Autodesk Inventor part; units mm, degrees
ref_plane "YZ Plane" through (0, 0, 0) normal (1, 0, 0) x (0, 1, 0)
ref_plane "XZ Plane" through (0, 0, 0) normal (0, 1, 0) x (-1, 0, 0)
ref_plane "XY Plane" through (0, 0, 0) normal (0, 0, 1) x (1, 0, 0)
sketch "Skizze1" plane through (0, 0, 0) normal (0, 0, 1) x (1, 0, 0)
  line L0 (-210, 0) -> (210, 0)
  line L1 (0, -168) -> (0, 168)
  ellipse E0 centre (0, 0) end of major axis (-150, 0) minor radius 120
  line L2 (0, 120) -> (0, -120) construction
  line L3 (-150, 0) -> (150, 0) construction
  dimension "d0" = 300
  dimension "d1" = 240
extrude "Extrusion1" add sketch "Skizze1" along normal blind 10
sketch "Skizze2" plane through (0, 0, 10) normal (0, 0, 1) x (1, 0, 0)
  ellipse E0 centre (0, 0) end of major axis (-150, 0) minor radius 120
  line L0 (0, -168) -> (0, 168)
  line L1 (-210, 0) -> (210, 0)
  line L2 (-131.5, 0) -> (131.5, 0)
  line L3 (0, 101.5) -> (0, -101.5)
  ellipse E1 centre (0, 0) end of major axis (-131.5, 0) minor radius 101.5
  line L4 (0, 0) -> (-105.3012, -60.7957) construction
  line L5 (0, 0) -> (105.3012, -60.7957) construction
  ellipse E2 centre (0, 0) end of major axis (118.5, 0) minor radius 88.5
  line L6 (0, 0) -> (80.349, 80.349) construction
  line L7 (80.349, 80.349) -> (73.764, 69.2632)
  line L8 (67.3414, 73.0783) -> (84.3123, 62.9974)
  arc A0 (94.9826, -52.9176) -> (105.1165, -60.6891) centre (99.5391, -57.469) ccw
  arc A1 (-105.1165, -60.6891) -> (-94.9826, -52.9176) centre (-99.5391, -57.469) ccw
  point P0 (0, 120)
  point P1 (150, 0)
  point P2 (-150, 0)
  point P3 (0, -120)
  point P4 (118.5, 0)
  point P5 (-96, 0)
  point P6 (0, 88.5)
  point P7 (-104.0928, -62.0231)
  point P8 (104.0928, -62.0231)
  dimension "d7" = 18.5
  dimension "d8" = 18.5
  dimension "d9" = 31.5
  dimension "d10" = 31.5
  dimension "d11" = 45
  dimension "d12" = 90
  dimension "d13" = 12.8941
  dimension "d14" = 30
  dimension "d15" = 30
extrude "Extrusion2" cut sketch "Skizze2" against normal through all contours E1 L0 E2 L1 | L1 E2 A1 E1 | E1 L7 E2 L0 | E1 A0 E2 L1 | L1 E2 L7 E1
sketch "Skizze4" plane through (0, 0, 10) normal (0, 0, 1) x (1, 0, 0)
  circle A0 centre (0, 0) radius 27.5
extrude "Extrusion4" cut sketch "Skizze4" against normal through all
sketch "Skizze5" plane through (0, 0, 10) normal (0, 0, 1) x (1, 0, 0)
  circle A0 centre (44.6817, 16.1402) radius 2.2
  circle A1 centre (81.576, 6.678) radius 2.2
  circle A2 centre (81.1696, 28.4843) radius 2.2
  circle A3 centre (34.1537, 26.537) radius 2.2
  circle A4 centre (-1.9423, 37.1246) radius 2.2
  circle A5 centre (-37.5824, 25.8884) radius 2.2
  circle A6 centre (-46.0331, 14.7062) radius 2.2
  circle A7 centre (-82.7479, 3.0545) radius 2.1998
  circle A8 centre (-82.7419, 24.8643) radius 2.1999
  circle A9 centre (-49.2342, 62.6033) radius 2.2
  circle A10 centre (-27.4241, 62.5973) radius 2.2
  circle A11 centre (-13.5942, 73.8395) radius 2.2001
  circle A12 centre (8.2159, 73.8333) radius 2.2
  circle A13 centre (22.5018, 63.2519) radius 2.2
  circle A14 centre (44.3119, 63.2458) radius 2.2
  point P0 (0, 0)
hole "Bohrung1" at (81.576, 6.678, 10) at (81.1696, 28.4843, 10) at (44.6817, 16.1402, 10) at (34.1537, 26.537, 10) at (-1.9423, 37.1246, 10) at (8.2159, 73.8333, 10) at (-13.5942, 73.8395, 10) at (22.5018, 63.2519, 10) at (44.3119, 63.2458, 10) at (-27.4241, 62.5973, 10) at (-49.2342, 62.6033, 10) at (-37.5824, 25.8884, 10) at (-46.0331, 14.7062, 10) at (-82.7479, 3.0545, 10) at (-82.7419, 24.8643, 10) direction (0, 0, -1) diameter 3.242 end through all
sketch "Skizze6" plane through (0, 0, 0) normal (0, 0, -1) x (-1, 0, 0)
  point P0 (0, 0)
properties part number "24_0497_002" material "LCP-Kunststoff"
Can you work these out from the model? Positions are in its coordinate system, mm. Give positions to 0.01 mm unless a question says otherwise; leave off trailing zeros. Use one line per item in the form item = value. Start each with the question number.
(1) I want a section at A-A, the plane z = 4.5. State how many separate pieces and enclosed holes the cut face has, and give its area (3 significant figures).
(2) Please list where these lines run through material, in increasing order: line 1 (X direction, y = -42.5, z = 8.5); line 2 (X direction, y = -3.5, z = 6); line 3 (Y direction, x = -101, z = 6.5).
(3) Thinking about a two-plate mould opening in X: for faces 1 (the cylindrical face through (-5.961, -26.846, 5.07)), 2 (the flat face through (31, 2, 0)), which applies, released by +X, released by -X, zero draft, split by the parting line, or undercut?
(4) I'm going to push flat-ended pins straight in: P1, Ø1, axis at x = 27.5, z = 7.5, coming from the +Y side; P2, Ø5, axis at x = -26.5, z = 8.5, coming from the -Y side; P3, Ø6, axis at y = -29.5, z = 7.5, coming from the +X side. Where does each tip first touch, or does it pass through?
Worked out:
q1.separate_pieces = 1
q1.enclosed_holes = 17
q1.area = 47,800 mm²
q2.line_1 = -140.28 to -119.42, -103.94 to 103.94, 119.42 to 140.28
q2.line_2 = -149.94 to -131.42, -118.41 to -27.28, 27.28 to 118.41, 131.42 to 149.94
q2.line_3 = -88.72 to -63.74, -46.29 to 46.29, 65 to 88.72
q3.face_1 = undercut
q3.face_2 = zero draft
q4.P1 = 118.04
q4.P2 = -118.45
q4.P3 = 146.3
